Print and shaded views of the part. All mm, measured from the part's lowest x, y and z. Round coordinates to 2 decimals unless told otherwise and drop trailing zeros. Loops run counter-clockwise (first coordinate to the right, second up) from the corner with the lowest first, then second, coordinate; pieces in that order, holes last. Notation, with made-up numbers: (-7.5, -27) - (48.5, -27) arc R20 ccw to (48.5, -8) - close; hole circle Ø1 at (37.25, 47.5). An arc over 180 degrees is marked (long way). Use one line per item in the form item = value. Start each with the question number.
Q1. Saw through at C-C (x = 46). Give the cut face in (y, z) (1 decimal).
Q2. Mould opens along Z. For the marked faces 1, 2, 3 and 4 say: released by +Z, released by -Z, zero draft, split by the parting line, or undercut.
Q3. Saw through at D-D (y = 3.9). Give the cut face in (x, z) (1 decimal), then the cut area to 3 significant figures.
Q4. Saw through at A-A (x = 30.5). Give the cut face in (y, z).
Q5. Drill centre lines: line 1 (X direction, y = 2.25, z = 55.5) (1 decimal); line 2 (Z direction, x = 46.5, y = 3.75) (1 decimal); line 3 (X direction, y = 2.55, z = 53) (1 decimal). Where is each one in solid material? Low to high.
Q6. Saw through at B-B (z = 5.5). Give the cut face in (x, y), then the cut area to 3 significant figures.
Q7. Pin check, flat tips, straight feed: pin 1 (1 mm diameter, centred on y = 2.5, z = 32, fed in from -X); pin 2 (2 mm diameter, centred on y = 1.5, z = 8.5, fed in from +X); pin 3 (10.5 mm diameter, centred on x = 48.17, z = 48.18, fed in from -Y). Stop position of each tip, or through.
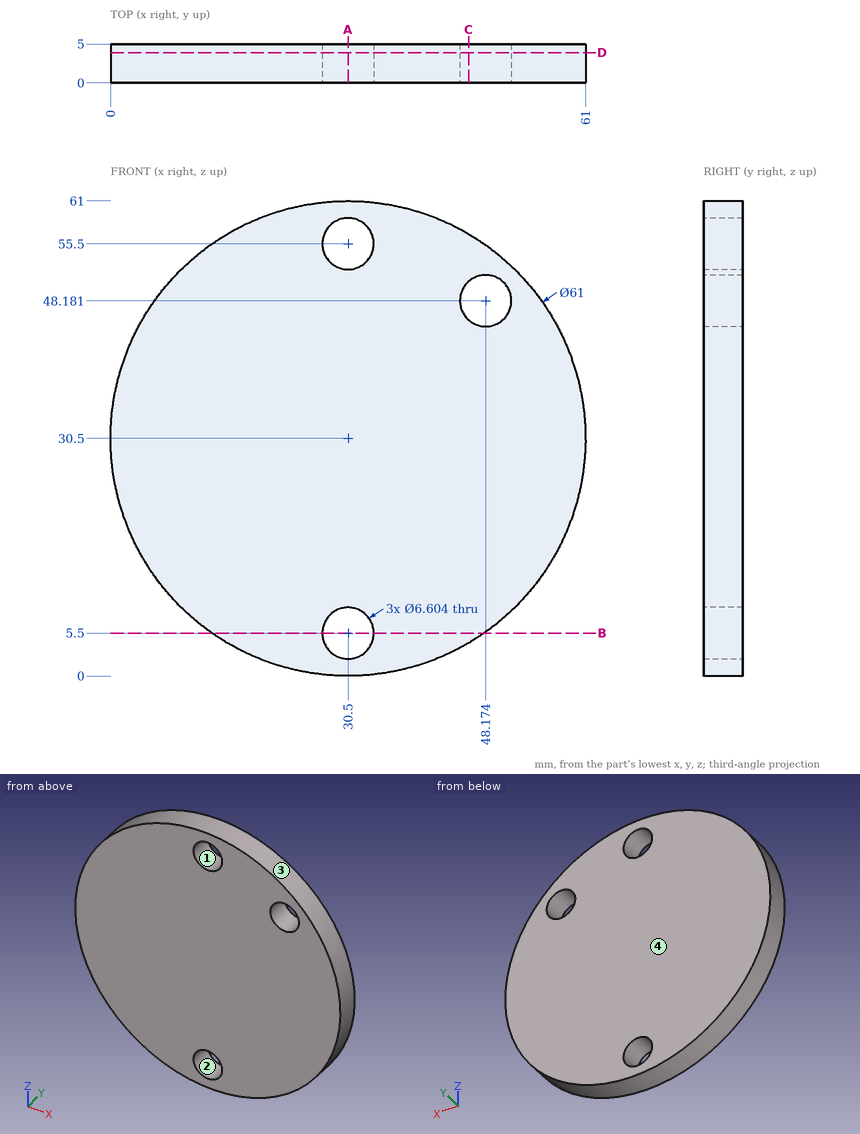
Report:
q1.outline = (0, 4.2) - (5, 4.2) - (5, 45.7) - (0, 45.7) - close; (0, 50.7) - (5, 50.7) - (5, 56.8) - (0, 56.8) - close
q2.face_1 = undercut
q2.face_2 = undercut
q2.face_3 = split by the parting line
q2.face_4 = zero draft
q3.outline = circle Ø61 at (30.5, 30.5); hole circle Ø6.6 at (30.5, 5.5); hole circle Ø6.6 at (30.5, 55.5); hole circle Ø6.6 at (48.2, 48.2)
q3.area = 2,820 mm²
q4.outline = (0, 0) - (5, 0) - (5, 2.2) - (0, 2.2) - close; (0, 8.8) - (5, 8.8) - (5, 52.2) - (0, 52.2) - close; (0, 58.8) - (5, 58.8) - (5, 61) - (0, 61) - close
q5.line_1 = 13 to 27.2, 33.8 to 48
q5.line_2 = 4.5 to 45.3, 51 to 56.5
q5.line_3 = 9.9 to 28.3, 32.7 to 51.1
q6.outline = (13.03, 0) - (27.2, 0) - (27.2, 5) - (13.03, 5) - close; (33.8, 0) - (47.97, 0) - (47.97, 5) - (33.8, 5) - close
q6.area = 142 mm²
q7.pin_1 = 0.02
q7.pin_2 = 52.62
q7.pin_3 = 0
